Check sheet for the modelled part. Datum: model origin and axes. Units: mm. Face numbers are marked on the shaded views. A direction names the side the tool comes from. Round coordinates to 2 decimals unless told otherwise and drop trailing zeros. Loops run counter-clockwise (first coordinate to the right, second up) from the corner with the lowest first, then second, coordinate; pieces in that order, holes last. Notation, with made-up numbers: (5.25, 60.5) -> (17.25, 60.5) arc R22 ccw to (17.25, 74.5) -> close; hole circle Ø9 at (-5, 4.25). An arc over 180 degrees is marked (long way). One line per question, with ' | ' between items.
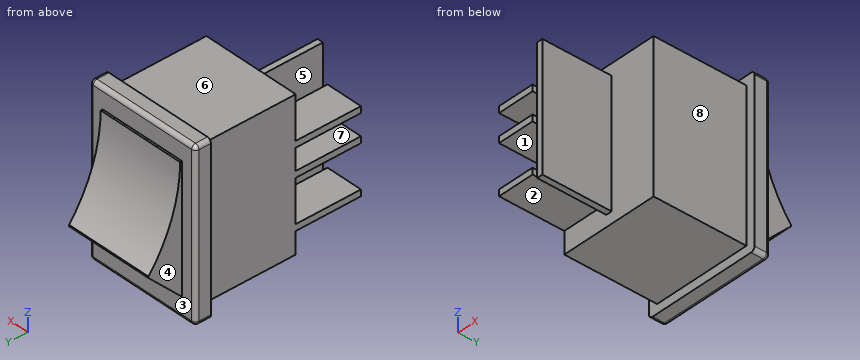
Autodesk Inventor part; units mm, degrees
ref_plane "YZ Plane" through (0, 0, 0) normal (1, 0, 0) x (0, 1, 0)
ref_plane "XZ Plane" through (0, 0, 0) normal (0, 1, 0) x (-1, 0, 0)
ref_plane "XY Plane" through (0, 0, 0) normal (0, 0, 1) x (1, 0, 0)
sketch "Sketch1" plane through (0, 0, 0) normal (0, 1, 0) x (-1, 0, 0)
  line L0 (7.495, 10.605) -> (-7.495, 10.605)
  line L1 (-7.495, 10.605) -> (-7.495, -10.605)
  line L2 (-7.495, -10.605) -> (7.495, -10.605)
  line L3 (7.495, -10.605) -> (7.495, 10.605)
  point P0 (0, 0)
  dimension "d0" = 14.99
  dimension "d1" = 7.495
  dimension "d2" = 21.21
  dimension "d3" = 10.605
extrude "Extrusion1" add sketch "Sketch1" against normal blind 2.03
sketch "Sketch2" plane through (0, -2.03, 0) normal (0, -1, 0) x (1, 0, 0)
  line L0 (-6.35, 9.46) -> (6.35, 9.46)
  line L1 (6.35, 9.46) -> (6.35, -9.46)
  line L2 (6.35, -9.46) -> (-6.35, -9.46)
  line L3 (-6.35, -9.46) -> (-6.35, 9.46)
  point P0 (0, 0)
  dimension "d6" = 12.7
  dimension "d7" = 6.35
  dimension "d8" = 18.92
  dimension "d9" = 9.46
extrude "Extrusion2" add sketch "Sketch2" along normal blind 11.93
sketch "Sketch3" plane through (0, -13.96, 0) normal (0, -1, 0) x (1, 0, 0)
  line L0 (-0.38, -8) -> (0.38, -8)
  line L1 (0.38, -8) -> (0.38, 8)
  line L2 (0.38, 8) -> (-0.38, 8)
  line L3 (-0.38, 8) -> (-0.38, -8)
  point P0 (0, 0)
  dimension "d12" = 0.76
  dimension "d13" = 0.38
  dimension "d14" = 16
  dimension "d15" = 8
extrude "Extrusion3" add sketch "Sketch3" along normal blind 8.89
fillet "Fillet1" radius 0.5 8 edges at (7.495, -1.015, -10.605) (7.495, 0, 0) (7.495, -1.015, 10.605) (0, 0, 10.605) (-7.495, -1.015, 10.605) (-7.495, 0, 0) (-7.495, -1.015, -10.605) (0, 0, -10.605)
sketch "Sketch4" plane through (0, -13.96, 0) normal (0, -1, 0) x (1, 0, 0)
  line L0 (-1.6, -6.675) -> (-6.35, -6.675)
  line L1 (-6.35, -6.675) -> (-6.35, -5.865)
  line L2 (-6.35, -5.865) -> (-1.6, -5.865)
  line L3 (-1.6, -5.865) -> (-1.6, -6.675)
  line L4 (-1.6, -0.405) -> (-6.35, -0.405)
  line L5 (-6.35, -0.405) -> (-6.35, 0.405)
  line L6 (-6.35, 0.405) -> (-1.6, 0.405)
  line L7 (-1.6, 0.405) -> (-1.6, -0.405)
  line L8 (-1.6, 3.145) -> (-6.35, 3.145)
  line L9 (-6.35, 3.145) -> (-6.35, 3.955)
  line L10 (-6.35, 3.955) -> (-1.6, 3.955)
  line L11 (-1.6, 3.955) -> (-1.6, 3.145)
  line L12 (-6.35, 9.46) -> (-6.35, -9.46)
  point P0 (0, 0)
  dimension "d19" = 0
  dimension "d20" = 4.75
  dimension "d21" = 4.75
  dimension "d22" = 0.81
  dimension "d23" = 0.81
  dimension "d24" = 0.81
  dimension "d25" = 5.46
  dimension "d26" = 2.74
  dimension "d28" = 0.405
extrude "Extrusion4" add sketch "Sketch4" along normal blind 8.38
sketch "Sketch5" plane through (0, 0, 0) normal (0, 1, 0) x (1, 0, 0)
  line L0 (5.65, 8) -> (-5.65, 8)
  line L1 (-5.65, 8) -> (-5.65, -8)
  line L2 (-5.65, -8) -> (5.65, -8)
  line L3 (5.65, -8) -> (5.65, 8)
  point P0 (0, 0)
  dimension "d31" = 16
  dimension "d32" = 8
  dimension "d33" = 11.3
  dimension "d34" = 5.65
extrude "Extrusion5" add sketch "Sketch5" along normal blind 4.32
sketch "Sketch7" plane through (-5.65, 0, 8) normal (-1, 0, 0) x (0, 0, 1)
  circle A0 centre (0.1807, 19.0432) radius 18.7949
  point P0 (-8, 0)
extrude "Extrusion7" cut sketch "Sketch7" along normal through all both and the other way through all
chamfer "Chamfer1" distance 4.32 angle 45 1 edges at (0, 4.32, -8) measured on face at (1.8833, 2.88, -8)
properties part number "GRSV-4011-0137_RockerSwitch"
(1) Set-up check for the marked faces 4, 5, 6, 7 and 8: record each of +Z, -Z, +X, -X, +Y, -Y from which the full face is reachable in a straight line by a thin tool's end or side.
Answer:
face 4: +Z, -Z, -X, +Y | face 5: +Z, -Z, -Y | face 6: +Z, +X, -X, -Y | face 7: -X, -Y | face 8: +Z, -Z, +X, -Y
(2) Sectioned sample at B-B, the plane z = 1.5. Record the cut outline in (x, y) (3 decimals).
Answer:
outline: (-7.495, -2.03) -> (-6.35, -2.03) -> (-6.35, -13.96) -> (-0.38, -13.96) -> (-0.38, -22.85) -> (0.38, -22.85) -> (0.38, -13.96) -> (6.35, -13.96) -> (6.35, -2.03) -> (7.495, -2.03) -> (7.495, -0.5) arc R0.5 ccw to (6.995, 0) -> (5.65, 0) -> (5.65, 1.476) -> (-5.65, 1.476) -> (-5.65, 0) -> (-6.995, 0) arc R0.5 ccw to (-7.495, -0.5) -> close
(3) Go/stop test with flat-tipped pins: pin 1 (1.4 mm diameter, centred on x = -3.5, y = -17, fed in from +Z) (3 decimals); pin 2 (10 mm diameter, centred on y = -19, z = -0.5, fed in from -X); pin 3 (1.3 mm diameter, centred on y = 3, z = 2, fed in from -X); pin 4 (1.4 mm diameter, centred on x = -5, y = -20, fed in from -Z) (3 decimals). Record where each tip stops, or that it passes through.
Answer:
pin 1: stops at z = 3.955 | pin 2: stops at x = -6.35 | pin 3: passes through | pin 4: stops at z = -6.675
(4) Mould release check, pull along Z, two halves, no side actions. Record for the marked faces 1, 2 and 3: +Z half, -Z half, draft (parallel to the pull), parting line (faces both ways), or undercut.
Answer:
face 1: undercut | face 2: -Z half | face 3: draft
(5) Scan lines: probe 1 along Z at (x, y) = (-2.5, -14) (3 decimals); probe 2 along Z at (x, y) = (0.75, -11.5); probe 3 along X at (y, z) = (-15.75, -2.5). Record each from-to range of solid material in increasing order.
Answer:
probe 1: z = -6.675 to -5.865, -0.405 to 0.405, 3.145 to 3.955 | probe 2: z = -9.46 to 9.46 | probe 3: x = -0.38 to 0.38
(6) Sectioned sample at C-C, the plane y = -4. Record the cut outline in (x, z), and give its area (3 significant figures).
Answer:
outline: (-6.35, -9.46) -> (6.35, -9.46) -> (6.35, 9.46) -> (-6.35, 9.46) -> close | area: 240 mm2
